from build123d import *

# Parameters (mm, degrees)
ESQUISSE1_W           = 15
ESQUISSE1_H           = 48
ESQUISSE2_R           = 30
EXTRUSION1_DEPTH      = 15
D_GAGEMENT_M391_D     = 44
D_GAGEMENT_M391_DEPTH = 18
PER_AGE1_D            = 8
PER_AGE1_CBORE_D      = 16
PER_AGE1_CBORE_DEPTH  = 5
PER_AGE2_D            = 8
PER_AGE2_CBORE_D      = 16
PER_AGE2_CBORE_DEPTH  = 5
PER_AGE3_D            = 8
PER_AGE3_CBORE_D      = 16
PER_AGE3_CBORE_DEPTH  = 5
PER_AGE4_D            = 8
PER_AGE4_CBORE_D      = 16
PER_AGE4_CBORE_DEPTH  = 5
CHANFREIN1_SIZE       = 1


# Read off the part's stored shape, not the designer's step: Enlèvement de matière-épaissir1, Enlèvement de matière-épaissir2
with BuildPart() as part:
    # Esquisse1 → Révolution1 (revolve)
    with BuildSketch(Plane.XY, mode=Mode.PRIVATE) as r_volution1_sk:
        with Locations((22.5, 24)):
            Rectangle(ESQUISSE1_W, ESQUISSE1_H)
    revolve(r_volution1_sk.sketch.rotate(Axis((15, 0, 0), (1, 0, 0)), 270), axis=Axis((15, 0, 0), (1, 0, 0)))

    # Esquisse2 → Extrusion1 (add)
    with BuildSketch(Plane.ZY.offset(-15)):
        Circle(ESQUISSE2_R)
    extrude(amount=EXTRUSION1_DEPTH)

    # Dégagement M391
    with Locations(Plane.ZY):
        with Locations((0, 0)):
            Hole(D_GAGEMENT_M391_D / 2, depth=D_GAGEMENT_M391_DEPTH)

    # Enlèvement de matière-épaissir1 outline → Enlèvement de matière-épaissir1 (revolve, cut)
    with BuildSketch(Plane.YX):
        with BuildLine():
            Line((0, 18), (20, 18))
            ThreePointArc((20, 18), (18.828427125, 20.828427125), (16, 22))
            Line((16, 22), (0, 22))
            Line((0, 22), (0, 18))
        make_face()
    revolve(axis=Axis((0, 0, 0), (1, 0, 0)), mode=Mode.SUBTRACT)

    # Enlèvement de matière-épaissir2 outline → Enlèvement de matière-épaissir2 (revolve, cut)
    with BuildSketch(Plane.YX):
        with BuildLine():
            Line((0, 26), (20, 26))
            ThreePointArc((20, 26), (22.828427125, 27.171572875), (24, 30))
            Line((24, 30), (0, 30))
            Line((0, 30), (0, 26))
        make_face()
    revolve(axis=Axis((0, 0, 0), (1, 0, 0)), mode=Mode.SUBTRACT)

    # Perçage1 (through all)
    with Locations(Plane(origin=(30, 0, 0), x_dir=(0, 0, -1), z_dir=(1, 0, 0))):
        with Locations((-38, 0)):
            CounterBoreHole(PER_AGE1_D / 2, PER_AGE1_CBORE_D / 2, PER_AGE1_CBORE_DEPTH)

    # Perçage2 (through all)
    with Locations(Plane(origin=(30, 0, 0), x_dir=(0, 0, -1), z_dir=(1, 0, 0))):
        with Locations((0, -38)):
            CounterBoreHole(PER_AGE2_D / 2, PER_AGE2_CBORE_D / 2, PER_AGE2_CBORE_DEPTH)

    # Perçage3 (through all)
    with Locations(Plane(origin=(30, 0, 0), x_dir=(0, 0, -1), z_dir=(1, 0, 0))):
        with Locations((0, 38)):
            CounterBoreHole(PER_AGE3_D / 2, PER_AGE3_CBORE_D / 2, PER_AGE3_CBORE_DEPTH)

    # Perçage4 (through all)
    with Locations(Plane(origin=(30, 0, 0), x_dir=(0, 0, -1), z_dir=(1, 0, 0))):
        with Locations((38, 0)):
            CounterBoreHole(PER_AGE4_D / 2, PER_AGE4_CBORE_D / 2, PER_AGE4_CBORE_DEPTH)

    # Chanfrein1
    chanfrein1_edges = [part.edges().sort_by_distance(p)[0] for p in [
        (0, 0, 22),
        (0, 0, -30),
    ]]
    chamfer(chanfrein1_edges, length=CHANFREIN1_SIZE)


solid = part.part
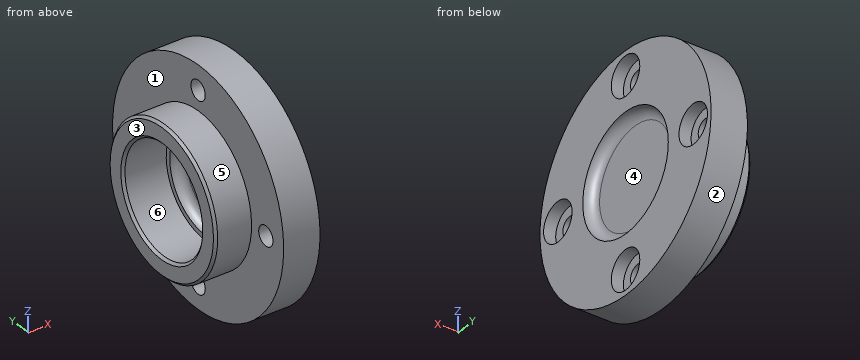
Input: part model. Units: mm. Frame: model coordinates. Face numbers are marked on the shaded views. A direction names the side the tool comes from. Coordinates: 2 decimals unless noted, no trailing zeros. Loops run counter-clockwise (first coordinate to the right, second up) from the corner with the lowest first, then second, coordinate; pieces in that order, holes last.
Q1. Material intervals for line 1 (Y direction, x = 14, z = 0); line 2 (Y direction, x = 25.25, z = 0); line 3 (Y direction, x = 28, z = -2), sorted ascending.
Q2. Set-up query: the marked faces 1 and 2. Return all of +Z, -Z, +X, -X, +Y, -Y with unobstructed straight access to the full face (end or side cutting, diameter ignored); none if empty.
Q3. Cut plane A-A (y = 36.5). Output: boundary loops of the cut face in (x, z), then the cut area to 3 significant figures.
Q4. Contact query for flat-ended pins moving along their axis: pin 1 (17.5 mm diameter, centred on y = -0.5, z = -39, fed in from +X); pin 2 (8 mm diameter, centred on x = 3.5, y = 22.5, fed in from +Z); pin 3 (3 mm diameter, centred on x = 23, z = 2.5, fed in from +Y); pin 4 (5 mm diameter, centred on y = 1.5, z = 36.5, fed in from +X). Output: stop coordinate, or through.
Q5. Draft query along Z for the marked faces 3, 4, 5 and 6. Return one class per face: +Z half, -Z half, draft (parallel to the pull), parting line (faces both ways), or undercut.
Q6. Cut plane B-B (z = 0). Give the number of separate pieces and of enclosed holes in the cut face, then the cut area to 3 significant figures.
Q7. Cut plane C-C (x = 12.75). Output: boundary loops of the cut face in (y, z).
Q8. Cut plane D-D (z = -38.5). Output: boundary loops of the cut face in (x, y).
Working result:
1. line 1: y = -30 to -22, 22 to 30
1. line 2: y = -48 to -46, -30 to 30, 46 to 48
1. line 3: y = -47.96 to -45.75, -30.25 to -23.38, 23.38 to 30.25, 45.75 to 47.96
2. face 1: -X
2. face 2: +X, -X
3. outline: (15, -31.17) - (30, -31.17) - (30, -7.86) - (25, -7.86) - (25, -3.71) - (15, -3.71) - close; (15, 3.71) - (25, 3.71) - (25, 7.86) - (30, 7.86) - (30, 31.17) - (15, 31.17) - close
3. area: 782 mm2
4. pin 1: stops at x = 30
4. pin 2: stops at z = 23.62
4. pin 3: stops at y = 47.99
4. pin 4: stops at x = 25
5. face 3: draft
5. face 4: undercut
5. face 5: parting line
5. face 6: undercut
6. separate pieces: 3
6. enclosed holes: 0
6. area: 888 mm2
7. outline: circle Ø60 at (0, 0); hole circle Ø44 at (0, 0)
8. outline: (15, -28.67) - (30, -28.67) - (30, -7.98) - (25, -7.98) - (25, -3.97) - (15, -3.97) - close; (15, 3.97) - (25, 3.97) - (25, 7.98) - (30, 7.98) - (30, 28.67) - (15, 28.67) - close
